Build history of the part. All positions in model axes, mm. A direction names the side the tool comes from. Give positions to 0.01 mm unless a question says otherwise; leave off trailing zeros. Write each loop counter-clockwise with the first axis right and the second up, starting at its lowest first coordinate (ties: lowest second). Pieces come first, ordered by that corner, then holes. Notation, with made-up numbers: (84.5, -25) -> (126.5, -25) arc R33 cw to (126.5, 4) -> close; hole circle Ø2 at (14.5, -40). An arc over 180 degrees is marked (long way). Put each result on its own line as item: value. Start each with the question number.
Item 1: Slice it at C-C, the plane x = -139.7. List the corners of the cut face in (y, z), plus the area to 3 significant figures.
Item 2: Slice it at B-B, the plane x = 0. List the corners of the cut face in (y, z), plus the area to 3 significant figures.
Item 3: Flat gauge pins, fed straight in: pin 1 Ø15 at (x, z) = (-63.5, 0) entering from +Y; pin 2 Ø6 at (y, z) = (-6.5, -8.5) entering from +X; pin 3 Ø5 at (x, y) = (-60.5, -9.5) entering from -Z; pin 4 Ø4 at (x, y) = (-143, -4) entering from +Z. Where does each tip first touch, or does it go through?
Item 4: Slice it at A-A, the plane y = -4.25. Give the number of separate pieces and of enclosed holes in the cut face, plus the area to 3 significant figures.
Item 5: Two-plate mould, pull along Z, no slides. Class faces 1 (the cylindrical face through (-17.219, -6.439, 11.108)), 2 (the cylindrical face through (-220.443, -6.439, -1.431)), 3 (the cylindrical face through (-287.342, -6.439, -0.209)), 4 (the flat face through (-168, -12.7, 5)): pulls with the +Z half, pulls with the -Z half, needs draft (parallel to the pull), parting line crosses it, or undercut.
Item 6: Slice it at D-D, the plane x = -278. List the corners of the cut face in (y, z), plus the area to 3 significant figures.
Item 7: Tool access for faces 5 (the cylindrical face through (-312.855, -6.439, -11.057)), 6 (the cylindrical face through (-93.3, -6.44, 1.82)), 7 (the cylindrical face through (-312.981, -6.439, 11.108)): list every direction of +Z, -Z, +X, -X, +Y, -Y with a clear straight run to the whole face (end or side of a thin tool).
Item 8: Drill centre lines: line 1 along X through (y, z) = (-6, -8); line 2 along Z through (x, y) = (-190.5, -4.5); line 3 along X through (y, z) = (-7.25, -9). Where is each one in solid material? Low to high.
```python
from build123d import *

# Parameters (mm, degrees)
F0_R     = 12.7
F1_DEPTH = 12.7
F2_D     = 9.525
F3_R     = 12.7


with BuildPart() as f1:
    # F0 (on Front) → F1 (new body)
    with BuildSketch(Plane.XZ):
        with BuildLine():
            Line((-314.085507, -10.16), (-16.114493, -10.16))
            ThreePointArc((-16.114493, -10.16), (19.05, 0), (-16.114493, 10.16))
            Line((-16.114493, 10.16), (-314.085507, 10.16))
            ThreePointArc((-314.085507, 10.16), (-349.25, 0), (-314.085507, -10.16))
        make_face()
        with Locations((-330.2, 0)):
            Circle(F0_R, mode=Mode.SUBTRACT)
        Circle(F0_R, mode=Mode.SUBTRACT)
    extrude(amount=F1_DEPTH)

    # F2 (through all)
    with Locations(Plane(origin=(0, 0, 0), x_dir=(1, 0, 0), z_dir=(0, 1, 0))):
        with Locations((-292.1, 0), (-266.7, 0), (-241.3, 0), (-215.9, 0), (-190.5, 0), (-165.1, 0), (-139.7, 0), (-114.3, 0), (-88.9, 0), (-63.5, 0), (-38.1, 0)):
            Hole(F2_D / 2)

    # F3
    f3_edges = [f1.edges().sort_by_distance(p)[0] for p in [
        (-314.085507, -6.35, -10.16),
        (-16.114493, -6.35, -10.16),
        (-16.114493, -6.35, 10.16),
        (-314.085507, -6.35, 10.16),
    ]]
    fillet(f3_edges, radius=F3_R)


solid = f1.part
```
Values follow:
1. outline: (-12.7, -10.16) -> (0, -10.16) -> (0, -4.76) -> (-12.7, -4.76) -> close; (-12.7, 4.76) -> (0, 4.76) -> (0, 10.16) -> (-12.7, 10.16) -> close
1. area: 137 mm2
2. outline: (-12.7, -19.05) -> (0, -19.05) -> (0, -12.7) -> (-12.7, -12.7) -> close; (-12.7, 12.7) -> (0, 12.7) -> (0, 19.05) -> (-12.7, 19.05) -> close
2. area: 161 mm2
3. pin 1: y = 0
3. pin 2: x = 18.24
3. pin 3: z = -10.16
3. pin 4: z = 10.16
4. separate pieces: 1
4. enclosed holes: 13
4. area: 6,470 mm2
5. face 1: pulls with the +Z half
5. face 2: undercut
5. face 3: undercut
5. face 4: needs draft
6. outline: (-12.7, -10.16) -> (0, -10.16) -> (0, 10.16) -> (-12.7, 10.16) -> close
6. area: 258 mm2
7. face 5: -Z, +Y, -Y
7. face 6: +Y, -Y
7. face 7: +Z, +Y, -Y
8. line 1: -347.49 to -340.06, -320.34 to -9.86, 9.86 to 17.29
8. line 2: -10.16 to -4.76, 4.76 to 10.16
8. line 3: -346.99 to -339.16, -321.24 to -8.96, 8.96 to 16.79
